Can you work these out from the model? Positions are in its coordinate system, mm. A direction names the side the tool comes from. Round coordinates to 2 decimals unless told otherwise and drop trailing zeros. Loops run counter-clockwise (first coordinate to the right, second up) from the corner with the lowest first, then second, coordinate; pieces in that order, holes last.
```python
from build123d import *

# Parameters (mm, degrees)
SALIENTE_EXTRUIR1_DEPTH    = 3
CORTAR_EXTRUIR5_DEPTH      = 104
CORTAR_EXTRUIR5_DEPTH_BACK = 142
CROQUIS1_5_W               = 25
CROQUIS1_5_H               = 80
CROQUIS2_W                 = 3
CROQUIS2_H                 = 50
SALIENTE_EXTRUIR2_DEPTH    = 30
CROQUIS3_R                 = 4.95
CROQUIS3_R_2               = 2.5
CROQUIS3_W                 = 6.5
CROQUIS3_H                 = 22.5
CORTAR_EXTRUIR6_DEPTH      = 30
CROQUIS4_R                 = 3.25
CORTAR_EXTRUIR7_DEPTH      = 1.5
CROQUIS5_R                 = 3.25
CORTAR_EXTRUIR8_DEPTH      = 3
REDONDEO11_R               = 15
REDONDEO12_START           = -65
REDONDEO12_DEPTH           = 130
REDONDEO12_2_DEPTH         = 3
REDONDEO12_START_2         = 62
REDONDEO12_3_DEPTH         = 3
REDONDEO13_R               = 15
CROQUIS7_R                 = 3
CROQUIS7_R_2               = 1.5
SALIENTE_EXTRUIR4_DEPTH    = 3.5
REDONDEO14_R               = 1
CROQUIS10_R                = 1.5
CORTAR_EXTRUIR11_DEPTH     = 3.5
CROQUIS6_R                 = 3.5
CROQUIS6_R_2               = 2.25
CORTAR_EXTRUIR12_DEPTH     = 1.5


with BuildPart() as part:
    # Croquis1 → Saliente-Extruir1 (new body)
    with BuildSketch(Plane(origin=(0, 0, 0), x_dir=(1, 0, 0), z_dir=(0, 1, 0))):
        Polygon((-90, 85), (-90, -85), (90, -85), (90, 85), (40.810665128, 108.620102865), (-39.189334872, 108.620102865), align=None)
    extrude(amount=SALIENTE_EXTRUIR1_DEPTH)

    # Croquis1<5> → Cortar-Extruir5 (cut, two sides: drawn at the far end of the back side and taken through both)
    with BuildSketch(Plane(origin=(0, 0, 0), x_dir=(1, 0, 0), z_dir=(0, 1, 0)).offset(-CORTAR_EXTRUIR5_DEPTH_BACK)):
        with Locations((-77.5, -45)):
            Rectangle(CROQUIS1_5_W, CROQUIS1_5_H)
        with Locations((77.5, -45)):
            Rectangle(CROQUIS1_5_W, CROQUIS1_5_H)
    extrude(amount=CORTAR_EXTRUIR5_DEPTH + CORTAR_EXTRUIR5_DEPTH_BACK, mode=Mode.SUBTRACT)

    # Croquis2 → Saliente-Extruir2 (add)
    with BuildSketch(Plane(origin=(0, 3, 0), x_dir=(1, 0, 0), z_dir=(0, 1, 0))):
        with Locations((-63.5, -30)):
            Rectangle(CROQUIS2_W, CROQUIS2_H)
    saliente_extruir2 = extrude(amount=SALIENTE_EXTRUIR2_DEPTH)

    # Croquis3 → Cortar-Extruir6 (cut)
    with BuildSketch(Plane.ZY.offset(65)):
        with Locations((40.353471705, 14.22)):
            Circle(CROQUIS3_R)
        with Locations((29.103471705, 14.22)):
            Circle(CROQUIS3_R_2)
        with Locations((8.25, 21.75)):
            Rectangle(CROQUIS3_W, CROQUIS3_H)
    cortar_extruir6 = extrude(amount=-CORTAR_EXTRUIR6_DEPTH, mode=Mode.SUBTRACT)

    # Simetría2: Saliente-Extruir2 across plane
    add(saliente_extruir2.mirror(Plane(origin=(0, 0, 0), x_dir=(0, 0, 1), z_dir=(1, 0, 0))))

    # Simetría3: Cortar-Extruir6 across plane
    add(cortar_extruir6.mirror(Plane(origin=(0, 0, 0), x_dir=(0, 0, 1), z_dir=(1, 0, 0))), mode=Mode.SUBTRACT)

    # Croquis4 → Cortar-Extruir7 (cut)
    with BuildSketch(Plane.XZ):
        with Locations(Location((-83.676954094, -80.966503939, 0), (0, 0, 270))):
            Circle(CROQUIS4_R)
    cortar_extruir7 = extrude(amount=-CORTAR_EXTRUIR7_DEPTH, mode=Mode.SUBTRACT)

    # Simetría4: Cortar-Extruir7 across plane
    add(cortar_extruir7.mirror(Plane(origin=(0, 0, 0), x_dir=(0, 0, 1), z_dir=(1, 0, 0))), mode=Mode.SUBTRACT)

    # Croquis5 → Cortar-Extruir8 (cut)
    with BuildSketch(Plane(origin=(0, 0, 0), x_dir=(-1, 0, 0), z_dir=(0, -1, 0))):
        with Locations(Location((0, -79, 0), (0, 0, 90))):
            Circle(CROQUIS5_R)
    extrude(amount=-CORTAR_EXTRUIR8_DEPTH, mode=Mode.SUBTRACT)

    # Redondeo11
    # the kernel refuses this fillet: 15 mm, written as the material it adds along each edge
    with BuildSketch(Plane(origin=(-65, 3, 5), x_dir=(0, 0, -1), z_dir=(1, 0, 0))) as redondeo11_piece_1:
        with BuildLine():
            CenterArc((12.990381057, 15), REDONDEO11_R, 210, 60)
            Line((0, 7.5), (0, 0))
            Line((0, 0), (12.990381057, 0))
        make_face()
    extrude(amount=3)
    with BuildSketch(Plane(origin=(65, 3, 5), x_dir=(0, 0, -1), z_dir=(-1, 0, 0))) as redondeo11_piece_2:
        with BuildLine():
            CenterArc((12.990381057, -15), REDONDEO11_R, 90, 60)
            Line((0, -7.5), (0, 0))
            Line((0, 0), (12.990381057, 0))
        make_face()
    extrude(amount=3)

    # Redondeo12: read off the stored shape, not the designer's step
    # Redondeo12 outline → Redondeo12 (cut)
    with BuildSketch(Plane.YZ.offset(REDONDEO12_START)):
        with BuildLine():
            Line((33, 55), (18, 55))
            ThreePointArc((18, 55), (28.606601718, 50.606601718), (33, 40))
            Line((33, 40), (33, 55))
        make_face()
    extrude(amount=REDONDEO12_DEPTH, mode=Mode.SUBTRACT)

    # Redondeo12 2 outline → Redondeo12 2 (add)
    with BuildSketch(Plane.YZ.offset(REDONDEO12_START)):
        with BuildLine():
            Line((3, 55), (18, 55))
            ThreePointArc((18, 55), (7.393398282, 59.393398282), (3, 70))
            Line((3, 70), (3, 55))
        make_face()
    extrude(amount=REDONDEO12_2_DEPTH)

    # Redondeo12 3 outline → Redondeo12 3 (add)
    with BuildSketch(Plane.YZ.offset(REDONDEO12_START_2)):
        with BuildLine():
            Line((3, 55), (18, 55))
            ThreePointArc((18, 55), (7.393398282, 59.393398282), (3, 70))
            Line((3, 70), (3, 55))
        make_face()
    extrude(amount=REDONDEO12_3_DEPTH)

    # Redondeo13
    redondeo13_edges = [part.edges().sort_by_distance(p)[0] for p in [
        (63.5, 33, 11.5),
        (-63.5, 33, 11.5),
    ]]
    fillet(redondeo13_edges, radius=REDONDEO13_R)

    # Croquis7 → Saliente-Extruir4 (add)
    # profile 1 of 8: a face of its own
    with BuildSketch(Plane(origin=(0, 3, 0), x_dir=(1, 0, 0), z_dir=(0, 1, 0))):
        with Locations(Location((-31.3, -59, 0), (0, 0, 90))):
            Circle(CROQUIS7_R)
        with Locations(Location((-31.3, -59, 0), (0, 0, 270))):
            Circle(CROQUIS7_R_2, mode=Mode.SUBTRACT)
    # profile 2 of 8: a face of its own
    with BuildSketch(Plane(origin=(0, 3, 0), x_dir=(1, 0, 0), z_dir=(0, 1, 0))):
        with Locations(Location((16.94328658, -60.27, 0), (0, 0, 90))):
            Circle(CROQUIS7_R)
        with Locations(Location((16.94328658, -60.27, 0), (0, 0, 270))):
            Circle(CROQUIS7_R_2, mode=Mode.SUBTRACT)
    # profile 3 of 8: a face of its own
    with BuildSketch(Plane(origin=(0, 3, 0), x_dir=(1, 0, 0), z_dir=(0, 1, 0))):
        with Locations(Location((11.86328658, -8.2, 0), (0, 0, 90))):
            Circle(CROQUIS7_R)
        with Locations(Location((11.86328658, -8.2, 0), (0, 0, 270))):
            Circle(CROQUIS7_R_2, mode=Mode.SUBTRACT)
    # profile 4 of 8: a face of its own
    with BuildSketch(Plane(origin=(0, 3, 0), x_dir=(1, 0, 0), z_dir=(0, 1, 0))):
        with Locations(Location((-16.07671342, -8.2, 0), (0, 0, 90))):
            Circle(CROQUIS7_R)
        with Locations(Location((-16.07671342, -8.2, 0), (0, 0, 270))):
            Circle(CROQUIS7_R_2, mode=Mode.SUBTRACT)
    # profile 5 of 8: a face of its own
    with BuildSketch(Plane(origin=(0, 3, 0), x_dir=(1, 0, 0), z_dir=(0, 1, 0))):
        with Locations(Location((11.86328658, 16.8, 0), (0, 0, 90))):
            Circle(CROQUIS7_R)
        with Locations(Location((11.86328658, 16.8, 0), (0, 0, 270))):
            Circle(CROQUIS7_R_2, mode=Mode.SUBTRACT)
    # profile 6 of 8: a face of its own
    with BuildSketch(Plane(origin=(0, 3, 0), x_dir=(1, 0, 0), z_dir=(0, 1, 0))):
        with Locations(Location((11.86328658, 53.8, 0), (0, 0, 90))):
            Circle(CROQUIS7_R)
        with Locations(Location((11.86328658, 53.8, 0), (0, 0, 270))):
            Circle(CROQUIS7_R_2, mode=Mode.SUBTRACT)
    # profile 7 of 8: a face of its own
    with BuildSketch(Plane(origin=(0, 3, 0), x_dir=(1, 0, 0), z_dir=(0, 1, 0))):
        with Locations(Location((-25.63671342, 16.8, 0), (0, 0, 90))):
            Circle(CROQUIS7_R)
        with Locations(Location((-25.63671342, 16.8, 0), (0, 0, 270))):
            Circle(CROQUIS7_R_2, mode=Mode.SUBTRACT)
    # profile 8 of 8: a face of its own
    with BuildSketch(Plane(origin=(0, 3, 0), x_dir=(1, 0, 0), z_dir=(0, 1, 0))):
        with Locations(Location((-25.63671342, 53.8, 0), (0, 0, 90))):
            Circle(CROQUIS7_R)
        with Locations(Location((-25.63671342, 53.8, 0), (0, 0, 270))):
            Circle(CROQUIS7_R_2, mode=Mode.SUBTRACT)
    extrude(amount=SALIENTE_EXTRUIR4_DEPTH)

    # Redondeo14
    redondeo14_edges = [part.edges().sort_by_distance(p)[0] for p in [
        (-31.3, 3, 62),
        (16.94328658, 3, 63.27),
        (11.86328658, 3, 11.2),
        (-16.07671342, 3, 11.2),
    ]]
    fillet(redondeo14_edges, radius=REDONDEO14_R)

    # Croquis10 → Cortar-Extruir11 (cut)
    with BuildSketch(Plane.XZ.offset(-1.5)):
        with Locations(Location((-83.676954094, -80.966503939, 0), (0, 0, 270))):
            Circle(CROQUIS10_R)
    cortar_extruir11 = extrude(amount=-CORTAR_EXTRUIR11_DEPTH, mode=Mode.SUBTRACT)

    # Simetría5: Cortar-Extruir11 across plane
    add(cortar_extruir11.mirror(Plane(origin=(0, 0, 0), x_dir=(0, 0, 1), z_dir=(1, 0, 0))), mode=Mode.SUBTRACT)

    # Croquis6 → Cortar-Extruir12 (cut)
    # profile 1 of 2: a face of its own
    with BuildSketch(Plane.XZ):
        with Locations(Location((-13.189334872, -87.120102865, 0), (0, 0, 270))):
            Circle(CROQUIS6_R)
        with Locations(Location((-13.189334872, -87.120102865, 0), (0, 0, 270))):
            Circle(CROQUIS6_R_2, mode=Mode.SUBTRACT)
    # profile 2 of 2: a face of its own
    with BuildSketch(Plane.XZ):
        with Locations(Location((14.810665128, -87.120102865, 0), (0, 0, 270))):
            Circle(CROQUIS6_R)
        with Locations(Location((14.810665128, -87.120102865, 0), (0, 0, 270))):
            Circle(CROQUIS6_R_2, mode=Mode.SUBTRACT)
    extrude(amount=-CORTAR_EXTRUIR12_DEPTH, mode=Mode.SUBTRACT)


solid = part.part
```
(1) If I drill on line 1 (X direction, y = 4.85, z = -16.8); line 2 (X direction, y = 19, z = 50.5); line 3 (X direction, y = 4, z = 61), over which ranges is the centre line in solid material (lowest first)?
(2) Suppose I cut it at A-A (y = 14.22). Write out the boundary of the cut face in (x, z).
(3) For pin 1 (1.5 mm diameter, centred on y = 25.5, z = 20.5, fed in from -X); pin 2 (8 mm diameter, centred on x = -15, z = 11, fed in from -Y); pin 3 (6.5 mm diameter, centred on x = -31, z = 60, fed in from +Y); pin 4 (8 mm diameter, centred on y = 13.5, z = 7.5, fed in from +X), each with a flat end and sliding along its axis, tell me the tip position at first contact or that it passes through.
(4) Suppose I cut it at D-D (x = 49.5). Write out the boundary of the cut face in (y, z), then the cut area to 3 significant figures.
(5) Suppose I cut it at B-B (z = -3.5). Write out the boundary of the cut face in (x, y).
(6) Suppose I cut it at C-C (y = 30.5). Write out the boundary of the cut face in (x, z), then the cut area to 3 significant figures.
(7) Which directions (+Z, -Z, +X, -X, +Y, -Y) give clear straight access to the entire face, cutting with the end or side of a thin tool? Please do faces 4 (the cylindrical face through (-80.937, 0.74, -82.714)), 5 (the cylindrical face through (-22.71, 4.73, -16.15)), 6 (the flat face through (-62, 18, 32)), 7 (the cylindrical face through (-63.52, 5.06, -0.4)), 8 (the flat face through (65.75, 1.479, -96.645)).
(8) We'd pull the mould along Z, two halves only. Please class faces 1 (the cylindrical face through (63.52, 14.44, 35.41)), 2 (the flat face through (18, 6.5, 62)), 3 (the flat face through (-64.239, 1.479, -96.975)): released by +Z, released by -Z, zero draft, split by the parting line, or undercut.
Check result:
1. line 1: x = -28.64 to -27.14, -24.14 to -22.64, 8.86 to 10.36, 13.36 to 14.86
1. line 2: x = -65 to -62, 62 to 65
1. line 3: x = -65 to -62, -33.54 to -29.06, 14.03 to 15.63, 18.25 to 19.85, 62 to 65
2. outline: (-65, 11.5) - (-62, 11.5) - (-62, 26.6) - (-65, 26.6) - close; (-65, 31.6) - (-62, 31.6) - (-62, 35.4) - (-65, 35.4) - close; (-65, 45.3) - (-62, 45.3) - (-62, 55.48) - (-65, 55.48) - close; (62, 11.5) - (65, 11.5) - (65, 26.6) - (62, 26.6) - close; (62, 31.6) - (65, 31.6) - (65, 35.4) - (62, 35.4) - close; (62, 45.3) - (65, 45.3) - (65, 55.48) - (62, 55.48) - close
3. pin 1: stops at x = -65
3. pin 2: stops at y = 0
3. pin 3: stops at y = 6.5
3. pin 4: stops at x = 65
4. outline: (0, -104.45) - (3, -104.45) - (3, 85) - (0, 85) - close
4. area: 568 mm2
5. outline: (-90, 0) - (90, 0) - (90, 3) - (65, 3) - (65, 3.69) - (62, 3.69) - (62, 3) - (-62, 3) - (-62, 3.69) - (-65, 3.69) - (-65, 3) - (-90, 3) - close
6. outline: (-65, 18.21) - (-62, 18.21) - (-62, 48.29) - (-65, 48.29) - close; (62, 18.21) - (65, 18.21) - (65, 48.29) - (62, 48.29) - close
6. area: 180 mm2
7. face 4: -Y
7. face 5: +Y
7. face 6: +Z, -Z, +Y
7. face 7: -Z, +X, -X, +Y
7. face 8: -Z, +X, +Y, -Y
8. face 1: undercut
8. face 2: zero draft
8. face 3: released by -Z
